Geometry: final body of the model. Coordinates: model frame, mm. A direction names the side the tool comes from. Give positions to 0.01 mm unless a question says otherwise; leave off trailing zeros. Loops run counter-clockwise (first coordinate to the right, second up) from the corner with the lowest first, then second, coordinate; pieces in that order, holes last. Notation, with made-up numbers: M 59.5,-23 L 79.5,-23 A17 cw 79.5,1 Z; hole C -19.5,12 d2. An arc over 180 degrees is marked long. Put each result on its own line as item: value.
```python
from build123d import *

# Parameters (mm, degrees)
F1_DEPTH     = 50
F3_D         = 20.2
F5_DEPTH     = 25
F6_T1_DEPTH  = 50
F6_T6_DEPTH  = 50
F6_T13_DEPTH = 50
F6_T19_DEPTH = 50
F6_T26_DEPTH = 50
F6_T33_DEPTH = 50
F6_T36_DEPTH = 72.2096061325
F6_T38_DEPTH = 75
F7_T1_DEPTH  = 4.6205948456
F7_T3_DEPTH  = 14
F8_W         = 20
F8_H         = 16
F8_W_2       = 4
F8_H_2       = 15.2079220091
F9_DEPTH     = 40
F10_D        = 12
F10_DEPTH    = 37
F10_TIP      = 3.6051637142


# Not quite as in the source:
# - a fillet or chamfer that OpenCascade refuses, or shapes differently, is made with other operations: its cross-section is extruded or revolved along the edge and cut away or added
# - a feature names something its author has since deleted; it is built from what else it names


with BuildPart() as f1:
    # F0 (on Front) → F1 (new body)
    with BuildSketch(Plane.XZ):
        Polygon((0, 30), (0, 0), (4, 0), (4, 30), (-10.0149744916, 148.1428074388), (-14.0149744916, 148.1428074388), (-80.0149744916, 148.1428074388), (-80.0149744916, 324.1428074388), (-84.0149744916, 324.1428074388), (-84.0149744916, 144.1428074388), (-14.0149744916, 144.1428074388), align=None)
    extrude(amount=F1_DEPTH)

    # F3 (through all)
    with Locations(Plane.YZ.offset(4)):
        with Locations((-25, 15)):
            Hole(F3_D / 2)

    # F4 (on face) → F5 (cut)
    with BuildSketch(Plane.YZ.offset(-80.0149744916)):
        Polygon((-50, 324.1428074388), (-50, 236.1428074388), (-50, 199.9447409799), (-50, 195.9447409799), (-50, 194.2019151126), (-50, 156.2548764067), (-50, 152.2548764067), (-39.9857666554, 240.1486744376), (-30.4158440182, 324.1428074388), align=None)
        Polygon((0, 324.1428074388), (-15.2079220091, 324.1428074388), (-7.806897337, 240.2772722232), (0, 151.8125457081), (0, 244.1428074388), align=None)
        Polygon((-45.5760135212, 155.7661052017), (-45.9782811199, 152.2160466314), (-4.1864533227, 151.8125457081), (-4.5209163536, 155.6025507861), (-24.936375975, 172.1473690272), align=None)
        Polygon((-9.0844288508, 207.3145008204), (-10.8621816933, 227.4593051175), (-22.1599204596, 218.427607474), align=None)
        Polygon((-42.1400031958, 186.0892978758), (-45.0776405527, 160.1643048917), (-27.431660318, 174.1695633191), align=None)
        Polygon((-39.5929888388, 208.4884916623), (-26.7007793174, 218.6382363502), (-37.4004572752, 227.7320942228), align=None)
        Polygon((-22.2456820263, 174.2829185178), (-4.9311455022, 160.2511080648), (-7.2217303873, 186.2071257598), align=None)
        Polygon((-8.7363235607, 203.3699069618), (-24.3721529686, 216.6590929463), (-40.0940653957, 204.0905991656), (-40.7694266569, 198.1630294508), (-8.2490940623, 197.8488116452), align=None)
        Polygon((-41.6920664445, 190.0423920546), (-24.7411634004, 176.305272485), (-7.5520306119, 189.9499595352), (-7.9272601749, 194.2019151126), (-41.2207386286, 194.2019151126), align=None)
    extrude(amount=-F5_DEPTH, mode=Mode.SUBTRACT)

    # F6: fillet of radius 5 on 4 edges, made by hand

    # F6_s2 → F6_t1 (join)
    with BuildSketch(Plane.XZ):
        with BuildLine():
            ThreePointArc((-18.4386008144, 144.1428074388), (-15.1255005733, 142.8875860427), (-13.4758700562, 139.7521541558))
            Line((-13.4758700562, 139.7521541558), (-14.0149744916, 144.1428074388))
            Line((-14.0149744916, 144.1428074388), (-18.4386008144, 144.1428074388))
        make_face()
    extrude(amount=F6_T1_DEPTH)


with BuildPart() as f6_tool4:
    # F6_s5 → F6_t6 (new body)
    with BuildSketch(Plane.XZ):
        with BuildLine():
            ThreePointArc((-80.0149744916, 153.1428074388), (-78.5505083975, 149.6072735328), (-75.0149744916, 148.1428074388))
            Line((-75.0149744916, 148.1428074388), (-80.0149744916, 148.1428074388))
            Line((-80.0149744916, 148.1428074388), (-80.0149744916, 153.1428074388))
        make_face()
    extrude(amount=F6_T6_DEPTH)

    split(bisect_by=Plane(origin=(0, 13.2937308283, 1.1731544977), x_dir=(1, 0, 0), z_dir=(0, -0.9961286805, -0.0879070636)), keep=Keep.TOP)

    split(bisect_by=Plane(origin=(0, 1.465226283, 151.7579786298), x_dir=(1, 0, 0), z_dir=(0, 0.0096545698, 0.9999533936)), keep=Keep.TOP)

    split(bisect_by=Plane(origin=(0, 9.1396289593, 0.8065603975), x_dir=(1, 0, 0), z_dir=(0, 0.9961286805, 0.0879070636)), keep=Keep.TOP)


with BuildPart() as f1_1:
    add(f1.part)

    # F6_t3: union F6_tool4
    add(f6_tool4.part)


with BuildPart() as f6_tool11:
    # F6_s12 → F6_t13 (new body)
    with BuildSketch(Plane.XZ):
        with BuildLine():
            ThreePointArc((-80.0149744916, 153.1428074388), (-78.5505083975, 149.6072735328), (-75.0149744916, 148.1428074388))
            Line((-75.0149744916, 148.1428074388), (-80.0149744916, 148.1428074388))
            Line((-80.0149744916, 148.1428074388), (-80.0149744916, 153.1428074388))
        make_face()
    extrude(amount=F6_T13_DEPTH)

    split(bisect_by=Plane(origin=(0, 1.465226283, 151.7579786298), x_dir=(1, 0, 0), z_dir=(0, -0.0096545698, -0.9999533936)), keep=Keep.TOP)

    split(bisect_by=Plane(origin=(0, 9.1396289593, 0.8065603975), x_dir=(1, 0, 0), z_dir=(0, 0.9961286805, 0.0879070636)), keep=Keep.TOP)


with BuildPart() as f1_2:
    add(f1_1.part)

    # F6_t10: union F6_tool11
    add(f6_tool11.part)


with BuildPart() as f6_tool17:
    # F6_s18 → F6_t19 (new body)
    with BuildSketch(Plane.XZ):
        with BuildLine():
            ThreePointArc((-80.0149744916, 153.1428074388), (-78.5505083975, 149.6072735328), (-75.0149744916, 148.1428074388))
            Line((-75.0149744916, 148.1428074388), (-80.0149744916, 148.1428074388))
            Line((-80.0149744916, 148.1428074388), (-80.0149744916, 153.1428074388))
        make_face()
    extrude(amount=F6_T19_DEPTH)

    split(bisect_by=Plane(origin=(0, -62.4248064238, 7.0735387838), x_dir=(1, 0, 0), z_dir=(0, 0.9936412568, -0.1125924191)), keep=Keep.TOP)

    split(bisect_by=Plane(origin=(0, 1.465226283, 151.7579786298), x_dir=(1, 0, 0), z_dir=(0, -0.0096545698, -0.9999533936)), keep=Keep.TOP)

    split(bisect_by=Plane(origin=(0, 9.1396289593, 0.8065603975), x_dir=(1, 0, 0), z_dir=(0, -0.9961286805, -0.0879070636)), keep=Keep.TOP)


with BuildPart() as f1_3:
    add(f1_2.part)

    # F6_t16: union F6_tool17
    add(f6_tool17.part)


with BuildPart() as f6_tool24:
    # F6_s25 → F6_t26 (new body)
    with BuildSketch(Plane.XZ):
        with BuildLine():
            ThreePointArc((-80.0149744916, 153.1428074388), (-78.5505083975, 149.6072735328), (-75.0149744916, 148.1428074388))
            Line((-75.0149744916, 148.1428074388), (-80.0149744916, 148.1428074388))
            Line((-80.0149744916, 148.1428074388), (-80.0149744916, 153.1428074388))
        make_face()
    extrude(amount=F6_T26_DEPTH)

    split(bisect_by=Plane(origin=(0, -66.484199108, 7.5749176678), x_dir=(1, 0, 0), z_dir=(0, 0.9935718557, -0.1132032138)), keep=Keep.TOP)

    split(bisect_by=Plane(origin=(0, -62.4248064238, 7.0735387838), x_dir=(1, 0, 0), z_dir=(0, -0.9936412568, 0.1125924191)), keep=Keep.TOP)

    split(bisect_by=Plane(origin=(0, 1.465226283, 151.7579786298), x_dir=(1, 0, 0), z_dir=(0, 0.0096545698, 0.9999533936)), keep=Keep.TOP)


with BuildPart() as f1_4:
    add(f1_3.part)

    # F6_t23: union F6_tool24
    add(f6_tool24.part)


with BuildPart() as f6_tool31:
    # F6_s32 → F6_t33 (new body)
    with BuildSketch(Plane.XZ):
        with BuildLine():
            ThreePointArc((-80.0149744916, 153.1428074388), (-78.5505083975, 149.6072735328), (-75.0149744916, 148.1428074388))
            Line((-75.0149744916, 148.1428074388), (-80.0149744916, 148.1428074388))
            Line((-80.0149744916, 148.1428074388), (-80.0149744916, 153.1428074388))
        make_face()
    extrude(amount=F6_T33_DEPTH)

    split(bisect_by=Plane(origin=(0, -62.4248064238, 7.0735387838), x_dir=(1, 0, 0), z_dir=(0, -0.9936412568, 0.1125924191)), keep=Keep.TOP)

    split(bisect_by=Plane(origin=(0, 1.465226283, 151.7579786298), x_dir=(1, 0, 0), z_dir=(0, -0.0096545698, -0.9999533936)), keep=Keep.TOP)


with BuildPart() as f1_5:
    add(f1_4.part)

    # F6_t30: union F6_tool31
    add(f6_tool31.part)

    # F6_s37 → F6_t36 (cut)
    with BuildSketch(Plane.XZ.offset(-11.1048030662)):
        with BuildLine():
            ThreePointArc((-14.4568957181, 148.1428074388), (-11.1361304097, 146.8807905536), (-9.4917098577, 143.7318145454))
            Line((-9.4917098577, 143.7318145454), (-10.0149744916, 148.1428074388))
            Line((-10.0149744916, 148.1428074388), (-14.4568957181, 148.1428074388))
        make_face()
    extrude(amount=F6_T36_DEPTH, mode=Mode.SUBTRACT)

    # F6_s39 → F6_t38 (cut)
    with BuildSketch(Plane.XZ.offset(-12.5)):
        with BuildLine():
            ThreePointArc((-79.0149744916, 144.1428074388), (-82.5505083975, 145.6072735328), (-84.0149744916, 149.1428074388))
            Line((-84.0149744916, 149.1428074388), (-84.0149744916, 144.1428074388))
            Line((-84.0149744916, 144.1428074388), (-79.0149744916, 144.1428074388))
        make_face()
    extrude(amount=F6_T38_DEPTH, mode=Mode.SUBTRACT)

    # F7: fillet of radius 2 on 3 edges, made by hand

    # F7_s2 → F7_t1 (cut)
    with BuildSketch(Plane.YZ.offset(-84.2351683711)):
        with BuildLine():
            ThreePointArc((0, 151.7244681563), (-0.0019365973, 151.8124604227), (-0.007742639, 151.9002822835))
            Line((-0.007742639, 151.9002822835), (0, 151.8125457081))
            Line((0, 151.8125457081), (0, 151.7244681563))
        make_face()
    extrude(amount=F7_T1_DEPTH, mode=Mode.SUBTRACT)

    # F7_s4 → F7_t3 (cut)
    with BuildSketch(Plane.YZ.offset(-5)):
        with BuildLine():
            ThreePointArc((-50, 2), (-49.4142135624, 0.5857864376), (-48, 0))
            Line((-48, 0), (-50, 0))
            Line((-50, 0), (-50, 2))
        make_face()
        with BuildLine():
            ThreePointArc((0, 2), (-0.5857864376, 0.5857864376), (-2, 0))
            Line((-2, 0), (0, 0))
            Line((0, 0), (0, 2))
        make_face()
    extrude(amount=F7_T3_DEPTH, mode=Mode.SUBTRACT)

    # F8 (on face) → F9 (join)
    with BuildSketch(Plane.XY.offset(324.1428074388)):
        with Locations((-82.0149744916, -22.8118830136)):
            Rectangle(F8_W, F8_H)
        with Locations((-82.0149744916, -22.8118830136)):
            Rectangle(F8_W_2, F8_H_2, mode=Mode.SUBTRACT)
    extrude(amount=-F9_DEPTH)

    # F10
    with Locations(Plane.XY.offset(324.1428074388)):
        with Locations((-82.0149744916, -22.8118830136)):
            Hole(F10_D / 2, depth=F10_DEPTH)
            with Locations((0, 0, -(F10_DEPTH + F10_TIP / 2))):  # 118° drill point
                Cone(0, F10_D / 2, F10_TIP, mode=Mode.SUBTRACT)


solid = f1_5.part
```
Item 1: Line query: probe 1 along Z at (x, y) = (-28, -22); probe 2 along X at (y, z) = (-14.5, 231.5); probe 3 along Z at (x, y) = (-86, -18). Output: solid intervals per line, ascending. Write a range as [from, to].
Output values:
probe 1: [144.14, 148.14]
probe 2: [-84.01, -80.01]
probe 3: [284.14, 324.14]
Item 2: Pin query (flat end, axial travel): pin 1 Ø8 at (y, z) = (-35, 124) entering from +X; pin 2 Ø5 at (y, z) = (-22.5, 244) entering from -X (3 decimals); pin 3 Ø1 at (x, y) = (-23.5, -35) entering from +Z. Return the tip coordinate at first contact, or that it passes through.
Output values:
pin 1: x = -6.68
pin 2: x = -84.015
pin 3: z = 148.14
Item 3: Section A-A on z = 15. Output: boundary loops of the cut face in (x, y), then the cut area to 3 significant figures.
Output values:
outline: M 0,-50 L 4,-50 L 4,-35.1 L 0,-35.1 Z; M 0,-14.9 L 4,-14.9 L 4,0 L 0,0 Z
area: 119 mm²
Item 4: Mould query, pull axis X, two halves, no side actions, for faces 1 (the conical face through (-82.241, -23.829, 284.164)), 2 (the flat face through (-49, -25, 144.143)), 3 (the flat face through (4, -14, 15)). Classes: pulls with the +X half, pulls with the -X half, needs draft (parallel to the pull), parting line crosses it, or undercut.
Output values:
face 1: undercut
face 2: needs draft
face 3: pulls with the +X half
Item 5: Set-up query: faces 4 (the flat face through (-76, -23, 284.143)), 5 (the cylindrical face through (-76.02, -22.55, 305.38)), 6 (the flat face through (-72.015, -23, 304)), 7 (the flat face through (-88, -23, 284.143)), 8 (the flat face through (-81.987, -14.629, 180.328)). Return all of +Z, -Z, +X, -X, +Y, -Y with unobstructed straight access to the full face (end or side cutting, diameter ignored); none if empty.
Output values:
face 4: +X, +Y, -Y
face 5: +Z
face 6: +Z, +X, +Y, -Y
face 7: -Z, -X, +Y, -Y
face 8: +X, -X
Item 6: Section B-B on x = -58. Output: boundary loops of the cut face in (y, z), then the cut area to 3 significant figures.
Output values:
outline: M -50,144.14 L 0,144.14 L 0,148.14 L -50,148.14 Z
area: 200 mm²
Item 7: Section C-C on z = 137. Output: boundary loops of the cut face in (x, y), then the cut area to 3 significant figures.
Output values:
outline: M -13.14,-50 L -8.69,-50 L -8.69,0 L -13.14,0 Z
area: 222 mm²
